```python
from build123d import *

# Parameters (mm, degrees)
F0_W     = 88.9
F0_H     = 38.1
F1_DEPTH = 508
F3_DEPTH = 38.1


with BuildPart() as f1:
    # F0 (on Top) → F1 (new body)
    with BuildSketch(Plane.XY):
        with Locations((44.45, 19.05)):
            Rectangle(F0_W, F0_H)
    extrude(amount=F1_DEPTH)

    # F2 (on face) → F3 (cut, through all)
    with BuildSketch(Plane.XZ):
        Polygon((88.9, 508), (0, 508), (44.45, 502.92), align=None)
    extrude(amount=-F3_DEPTH, mode=Mode.SUBTRACT)


solid = f1.part
```
Geometry check sheet. Reference: the model listing, model coordinates, mm. A direction names the side the tool comes from. Give positions to 0.01 mm unless a question says otherwise; leave off trailing zeros. One line per question, with ' | ' between items.
Item 1: Scan lines: line 1 along Z through (x, y) = (44.5, 12.5); line 2 along Z through (x, y) = (37.5, 5). Record each from-to range of solid material in increasing order.
Determined:
line 1: 0 to 502.93 | line 2: 0 to 503.71
Item 2: Draft check along X on faces 1 (the flat face through (88.9, 19, 250)), 2 (the flat face through (44, 38.1, 250)), 3 (the flat face through (21.914, 18.783, 505.496)). Enter one of: released by +X, released by -X, zero draft, split by the parting line, or undercut.
Determined:
face 1: released by +X | face 2: zero draft | face 3: undercut
Item 3: Access from +Z, -Z, +X, -X, +Y, -Y to the whole of each face (thin tool, end or side, straight path). Record for faces 4 (the flat face through (44, 19, 0)), 5 (the flat face through (66.364, 18.783, 505.424)).
Determined:
face 4: -Z, +X, -X, +Y, -Y | face 5: +Z, +Y, -Y
